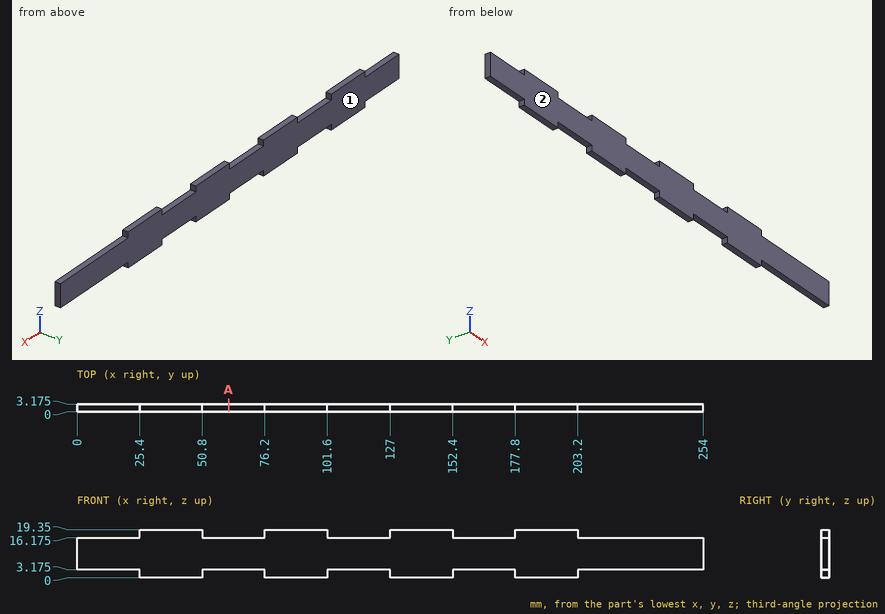
Design review of the part shown in the three views and the two pictorial views. Dimensions are in mm from the part's minimum x, y and z. Round coordinates to 2 decimals unless told otherwise and drop trailing zeros. Loops run counter-clockwise (first coordinate to the right, second up) from the corner with the lowest first, then second, coordinate; pieces in that order, holes last. Notation, with made-up numbers: M 24.25,-36 L 79.25,-36 A14 cw 79.25,-25 Z; hole C -11,61.5 d5. An arc over 180 degrees is marked long. Answer as a JSON object with one key per item and string values.
Item 1: Clearance check with flat-ended pins moving along their axes: P1, Ø1.6, axis at y = 2, z = 1, coming from the -X side; P2, Ø1, axis at x = 239.5, y = 2, coming from the -Z side (3 decimals); P3, Ø1, axis at y = 1.5, z = 2.5, coming from the +X side. State where each tip first meets the part, or that it passes through.
Check sheet entries:
{"P1": "x = 25.4", "P2": "z = 3.175", "P3": "x = 203.2"}
Item 2: The part is to be moulded in two halves that separate along Y. For the marked faces 1 and 2, say which applies: +Y half, -Y half, draft (parallel to the pull), parting line (faces both ways), or undercut.
Check sheet entries:
{"face 1": "+Y half", "face 2": "-Y half"}
Item 3: For line 1 along Z through (x, y) = (173.5, 1.75) (3 decimals), list the stretches that pass through material, from the lowest coordinate up.
Check sheet entries:
{"line 1": "3.175 to 16.175"}
Item 4: We need section A-A, the plane x = 61.5. State the section outline as (y, z) points (3 decimals), and give its area (3 significant figures).
Check sheet entries:
{"outline": "M 0,3.175 L 3.175,3.175 L 3.175,16.175 L 0,16.175 Z", "area": "41.3 mm2"}
